Work out the finished part from the listing and answer in its coordinate system (mm). A direction names the side the tool comes from. Coordinates: 2 decimals unless noted, no trailing zeros. Write each loop counter-clockwise with the first axis right and the second up, starting at its lowest first coordinate (ties: lowest second). Pieces come first, ordered by that corner, then holes. Notation, with made-up numbers: (-30.75, -0.5) - (15.25, -0.5) arc R21 cw to (15.25, 26.5) - close; hole circle Ø3 at (67, -1.75). An arc over 180 degrees is marked (long way). Use one line per item in the form item = value. Start each with the question number.
Item 1: For faces 4 (the flat face through (30, 311.15, -1)), 5 (the cylindrical face through (-60.47, 311.239, -46.367)), determine the directions among +Z, -Z, +X, -X, +Y, -Y from which every point of the face is accessible in a straight line to the end or side of a thin tool.
Item 2: A cutting plane is placed at C-C (y = 231.5). Write down the section's boundary in (x, z) (3 decimals), then the cut area to 3 significant figures.
Item 3: Determine the mould class of faces 1 (the cylindrical face through (-7.559, 150.266, 5.796)), 2 (the flat face through (-1, 317.5, -1)), 3 (the cylindrical face through (66.927, 308.019, 21.076)) for opening direction Z: released by +Z, released by -Z, zero draft, split by the parting line, or undercut.
Item 4: Consider probe 1 along Z at (x, y) = (0, 309); probe 2 along Y at (x, z) = (-7, 21); probe 3 along Y at (x, z) = (-33, 40). Determine where each line is inside the solid, lowest interval first.
Item 5: A cutting plane is placed at D-D (z = -44). Write down the section's boundary in (x, y), then the cut area to 3 significant figures.
Item 6: Given pin 1 (6 mm diameter, centred on y = 63, z = -8, fed in from -X); pin 2 (5 mm diameter, centred on x = 30.5, z = -35, fed in from -Y); pin 3 (8 mm diameter, centred on x = 15, y = 97, fed in from +Z), each flat-ended and moving along its own axis, determine where each tip first touches the part or whether it passes through.
from build123d import *

# Parameters (mm, degrees)
SKETCH1_R           = 9.525
BOSS_EXTRUDE1_DEPTH = 304.8
SKETCH2_R           = 28.2575
BOSS_EXTRUDE2_DEPTH = 6.35
SKETCH3_R           = 76.2
BOSS_EXTRUDE3_DEPTH = 6.35
SKETCH5_R           = 76.2
SKETCH5_R_2         = 70.1675
BOSS_EXTRUDE4_DEPTH = 6.35


with BuildPart() as part:
    # Sketch1 → Boss-Extrude1 (new body)
    with BuildSketch(Plane(origin=(0, 0, 0), x_dir=(1, 0, 0), z_dir=(0, 1, 0))):
        Circle(SKETCH1_R)
    extrude(amount=BOSS_EXTRUDE1_DEPTH)

    # Sketch2 → Boss-Extrude2 (add)
    with BuildSketch(Plane(origin=(0, 304.8, 0), x_dir=(1, 0, 0), z_dir=(0, 1, 0))):
        Circle(SKETCH2_R)
    extrude(amount=BOSS_EXTRUDE2_DEPTH)

    # Sketch3 → Boss-Extrude3 (add)
    with BuildSketch(Plane(origin=(0, 311.15, 0), x_dir=(1, 0, 0), z_dir=(0, 1, 0))):
        Circle(SKETCH3_R)
    extrude(amount=BOSS_EXTRUDE3_DEPTH)

    # Sketch5 → Boss-Extrude4 (add)
    with BuildSketch(Plane.XZ.offset(-311.15)):
        Circle(SKETCH5_R)
        Circle(SKETCH5_R_2, mode=Mode.SUBTRACT)
    extrude(amount=BOSS_EXTRUDE4_DEPTH)


solid = part.part
Answer:
q1.face_4 = -Y
q1.face_5 = +Y, -Y
q2.outline = circle Ø19.05 at (0, 0)
q2.area = 285 mm²
q3.face_1 = split by the parting line
q3.face_2 = zero draft
q3.face_3 = undercut
q4.probe_1 = -76.2 to -70.17, -28.26 to 28.26, 70.17 to 76.2
q4.probe_2 = 304.8 to 317.5
q4.probe_3 = 311.15 to 317.5
q5.outline = (-62.21, 304.8) - (-54.66, 304.8) - (-54.66, 311.15) - (54.66, 311.15) - (54.66, 304.8) - (62.21, 304.8) - (62.21, 317.5) - (-62.21, 317.5) - close
q5.area = 886 mm²
q6.pin_1 = -8.11
q6.pin_2 = 311.15
q6.pin_3 = through
